Could you check a few things on this model? Use its own coordinates, in mm. Give positions to 0.01 mm unless a question says otherwise; leave off trailing zeros. Write each loop counter-clockwise with the first axis right and the second up, starting at its lowest first coordinate (ties: lowest second). Pieces come first, ordered by that corner, then holes. Notation, with made-up numbers: (-18.5, -23) -> (9.5, -23) arc R16 cw to (9.5, -7) -> close; hole circle Ø2 at (-8.5, 70.5). An arc over 180 degrees is marked (long way). Write item = value, one per line. Start each with the question number.
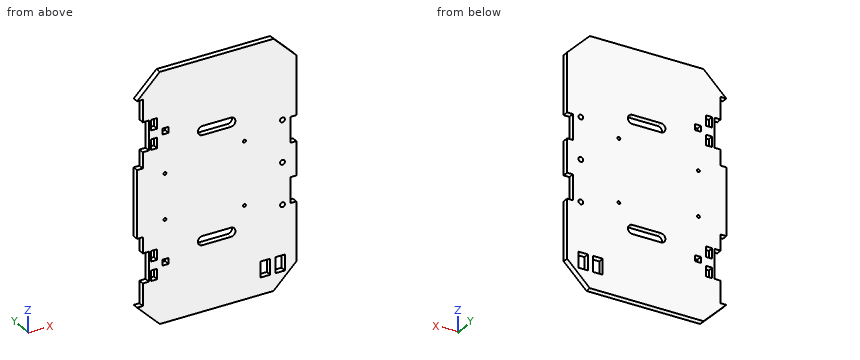
Autodesk Inventor part; units mm, degrees
ref_plane "YZ Plane" through (0, 0, 0) normal (1, 0, 0) x (0, 1, 0)
ref_plane "XZ Plane" through (0, 0, 0) normal (0, 1, 0) x (-1, 0, 0)
ref_plane "XY Plane" through (0, 0, 0) normal (0, 0, 1) x (1, 0, 0)
sketch "Sketch1" plane through (0, 0, 0) normal (0, 1, 0) x (-1, 0, 0)
  line L0 (145, 110) -> (-145, 110)
  line L1 (-145, 110) -> (-145, -110)
  line L2 (-145, -110) -> (145, -110)
  line L3 (145, -110) -> (145, 110)
  line L4 (145, 110) -> (-145, -110) construction
  line L5 (-145, 110) -> (145, -110) construction
  line L6 (105, -80.8333) -> (35, -80.8333)
  line L7 (35, -80.8333) -> (35, -115.8333)
  line L8 (35, -115.8333) -> (105, -115.8333)
  line L9 (105, -115.8333) -> (105, -80.8333)
  line L10 (105, -80.8333) -> (35, -115.8333) construction
  line L11 (35, -80.8333) -> (105, -115.8333) construction
  line L12 (-35, -115.8333) -> (-105, -115.8333)
  line L13 (-105, -115.8333) -> (-105, -80.8333)
  line L14 (-105, -80.8333) -> (-35, -80.8333)
  line L15 (-35, -80.8333) -> (-35, -115.8333)
  line L16 (-35, -115.8333) -> (-105, -80.8333) construction
  line L17 (-105, -115.8333) -> (-35, -80.8333) construction
  line L18 (0, 110) -> (0, -110) construction
  line L19 (5, -110) -> (5, 110)
  point P0 (0, 0)
  point P1 (70, -98.3333)
  point P2 (-70, -98.3333)
  point P3 (0, 0)
  point P4 (-105, -110)
  point P5 (-35, -110)
  point P6 (-15, -80.8333)
  point P7 (-55, -80.8333)
  point P8 (105, -110)
  point P9 (35, -110)
  dimension "d1" = 70
  dimension "d2" = 70
  dimension "d3" = 35
  dimension "d4" = 35
  dimension "d5" = 140
  dimension "d6" = 11.6667
  dimension "d7" = 220
  dimension "d8" = 290
  dimension "d34" = 140
extrude "Extrusion1" add sketch "Sketch1" along normal blind 5 contours L3 L2 L9 L6 L7 L19 L0 | L2 L7 L6 L9
sketch "Sketch5" plane through (0, 5, 0) normal (0, 1, 0) x (1, 0, 0)
  line L0 (-145, -110) -> (-5, -110) construction
  line L1 (-5, -110) -> (-5, 110) construction
  line L2 (-5, 110) -> (-145, 110) construction
  line L3 (-145, 110) -> (-145, -110) construction
  circle A0 centre (-120.5342, 20) radius 1.25
  circle A1 centre (-120.5342, -20) radius 1.25
  circle A2 centre (-50.5342, 28) radius 1.25
  circle A3 centre (-50.5342, -28) radius 1.25
  line L4 (-145, 0) -> (-5, 0) construction
  point P0 (0, 0)
  dimension "d35" = 56
  dimension "d36" = 40
  dimension "d37" = 70
  dimension "d38" = 2.5
  dimension "d39" = 2.5
extrude "Extrusion6" cut sketch "Sketch5" against normal through all
chamfer "Chamfer1" distance 20 angle 45 4 edges at (-145, 2.5, 110) (-145, 2.5, -110) (-5, 2.5, 110) (-5, 2.5, -110)
sketch "Sketch6" plane through (0, 5, 0) normal (0, 1, 0) x (1, 0, 0)
  circle A0 centre (-50.5342, -28) radius 1.25
  circle A1 centre (-50.5342, 28) radius 1.25
  circle A2 centre (-120.5342, -20) radius 1.25
  circle A3 centre (-120.5342, 20) radius 1.25
  line L0 (-25, 110) -> (-5, 90)
  line L1 (-25, 110) -> (-125, 110)
  line L2 (-145, 90) -> (-125, 110)
  line L3 (-145, 90) -> (-145, -90)
  line L4 (-125, -110) -> (-145, -90)
  line L5 (-125, -110) -> (-25, -110)
  line L6 (-5, -90) -> (-25, -110)
  line L7 (-5, -90) -> (-5, 90)
  line L8 (-145, 90) -> (-145, -90)
  line L9 (-5, 37.6) -> (-10, 37.6)
  line L10 (-10, 37.6) -> (-10, 15)
  line L11 (-10, 15) -> (-5, 15)
  line L12 (-5, 15) -> (-5, 37.6)
  line L13 (-5, 37.6) -> (-10, 15) construction
  line L14 (-10, 37.6) -> (-5, 15) construction
  line L15 (-5, -90) -> (-5, 90)
  line L16 (-87.5, 48) -> (-62.5, 48) construction
  line L17 (-87.5, 44) -> (-62.5, 44)
  line L18 (-62.5, 52) -> (-87.5, 52)
  arc A4 (-87.5, 52) -> (-87.5, 44) centre (-87.5, 48) ccw
  arc A5 (-62.5, 44) -> (-62.5, 52) centre (-62.5, 48) ccw
  line L19 (-145, 30) -> (-140, 30)
  line L20 (-140, 30) -> (-140, -30) construction
  line L21 (-140, -30) -> (-145, -30)
  line L22 (-145, -30) -> (-145, 30)
  line L23 (-145, 30) -> (-140, -30) construction
  line L24 (-140, 30) -> (-145, -30) construction
  line L25 (-140, 30) -> (-140, 95)
  line L26 (-140, -30) -> (-140, -95)
  line L27 (-145, 90) -> (-140, 90)
  point P0 (0, 0)
  point P1 (-7.5, 26.3)
  point P2 (-5, 15)
  point P3 (-5, 37.6)
  point P4 (-75, 48)
  point P5 (-75, 110)
  point P6 (-142.5, 0)
  point P7 (-145, 0)
  point P8 (-145, 0)
  dimension "d57" = 5
  dimension "d58" = 22.6
  dimension "d59" = 15
  dimension "d60" = 8
  dimension "d61" = 25
  dimension "d86" = 5
  dimension "d87" = 60
  dimension "d88" = 48
extrude "Extrusion7" cut sketch "Sketch6" against normal through all contours L7 L11 L10 L9 | L27 L25 L19 L3 | A4 L18 A5 L17
mirror "Mirror6" about plane through (0, 0, 0) normal (0, 0, 1) of "Extrusion7"
sketch "Sketch8" plane through (0, 5, 0) normal (0, 1, 0) x (1, 0, 0)
  circle A0 centre (-120.5342, 20) radius 1.25 construction
  circle A1 centre (-120.5342, -20) radius 1.25 construction
  circle A2 centre (-50.5342, 28) radius 1.25 construction
  circle A3 centre (-50.5342, -28) radius 1.25 construction
  line L0 (-87.5, 52) -> (-62.5, 52) construction
  arc A4 (-62.5, 44) -> (-62.5, 52) centre (-62.5, 48) ccw construction
  line L1 (-62.5, 44) -> (-87.5, 44) construction
  arc A5 (-87.5, 52) -> (-87.5, 44) centre (-87.5, 48) ccw construction
  line L2 (-87.5, -44) -> (-62.5, -44) construction
  arc A6 (-62.5, -52) -> (-62.5, -44) centre (-62.5, -48) ccw construction
  line L3 (-62.5, -52) -> (-87.5, -52) construction
  arc A7 (-87.5, -44) -> (-87.5, -52) centre (-87.5, -48) ccw construction
  line L4 (-125, -110) -> (-145, -90) construction
  line L5 (-125, -110) -> (-25, -110) construction
  line L6 (-5, -90) -> (-25, -110) construction
  line L7 (-5, -90) -> (-5, -37.6) construction
  line L8 (-5, -37.6) -> (-10, -37.6) construction
  line L9 (-10, -37.6) -> (-10, -15) construction
  line L10 (-10, -15) -> (-5, -15) construction
  line L11 (-5, -15) -> (-5, 15) construction
  line L12 (-5, 15) -> (-10, 15) construction
  line L13 (-10, 15) -> (-10, 37.6) construction
  line L14 (-10, 37.6) -> (-5, 37.6) construction
  line L15 (-5, 37.6) -> (-5, 90) construction
  line L16 (-25, 110) -> (-5, 90) construction
  line L17 (-25, 110) -> (-125, 110) construction
  line L18 (-145, 90) -> (-125, 110) construction
  line L19 (-145, 30) -> (-145, -30) construction
  line L20 (-23.3, 95) -> (-15, 95)
  line L21 (-15, 95) -> (-15, 81)
  line L22 (-15, 81) -> (-23.3, 81)
  line L23 (-23.3, 81) -> (-23.3, 95)
  line L24 (-23.3, 95) -> (-15, 81) construction
  line L25 (-15, 95) -> (-23.3, 81) construction
  line L26 (-36.3, 95) -> (-28, 95)
  line L27 (-28, 95) -> (-28, 81)
  line L28 (-28, 81) -> (-36.3, 81)
  line L29 (-36.3, 81) -> (-36.3, 95)
  line L30 (-36.3, 95) -> (-28, 81) construction
  line L31 (-28, 95) -> (-36.3, 81) construction
  line L32 (-132.6, -44.1) -> (-127.4, -44.1)
  line L33 (-127.4, -44.1) -> (-127.4, -53.3)
  line L34 (-127.4, -53.3) -> (-132.6, -53.3)
  line L35 (-132.6, -53.3) -> (-132.6, -44.1)
  line L36 (-132.6, -44.1) -> (-127.4, -53.3) construction
  line L37 (-127.4, -44.1) -> (-132.6, -53.3) construction
  line L38 (-132.6, -61.1) -> (-127.4, -61.1)
  line L39 (-127.4, -61.1) -> (-127.4, -70.3)
  line L40 (-127.4, -70.3) -> (-132.6, -70.3)
  line L41 (-132.6, -70.3) -> (-132.6, -61.1)
  line L42 (-132.6, -61.1) -> (-127.4, -70.3) construction
  line L43 (-127.4, -61.1) -> (-132.6, -70.3) construction
  line L44 (-117.4, -54.6) -> (-122.6, -54.6)
  line L45 (-122.6, -54.6) -> (-122.6, -59.8)
  line L46 (-122.6, -59.8) -> (-117.4, -59.8)
  line L47 (-117.4, -59.8) -> (-117.4, -54.6)
  line L48 (-117.4, -54.6) -> (-122.6, -59.8) construction
  line L49 (-122.6, -54.6) -> (-117.4, -59.8) construction
  line L50 (-130, -48.7) -> (-130, -65.7) construction
  line L51 (-140, -44.1) -> (-134.6, -44.1)
  line L52 (-134.6, -44.1) -> (-134.6, -70.3)
  line L53 (-134.6, -70.3) -> (-140, -70.3)
  line L54 (-140, -70.3) -> (-140, -44.1)
  line L55 (-140, -44.1) -> (-134.6, -70.3) construction
  line L56 (-134.6, -44.1) -> (-140, -70.3) construction
  line L57 (-140, 90) -> (-140, 30)
  line L58 (-140, 30) -> (-145, 30)
  line L59 (-145, -30) -> (-140, -30)
  line L60 (-140, -30) -> (-140, -90)
  circle A8 centre (-17.1, 0) radius 2.1
  circle A9 centre (-17.1, 37) radius 2.1
  circle A10 centre (-17.1, -37) radius 2.1
  point P0 (0, 0)
  point P1 (-19.15, 88)
  point P2 (-32.15, 88)
  point P3 (-120, -57.2)
  point P4 (-130, -57.2)
  point P5 (-137.3, -57.2)
  point P6 (-140, 95)
  point P7 (-140, -95)
  dimension "d63" = 14
  dimension "d64" = 8.3
  dimension "d65" = 14
  dimension "d66" = 8.3
  dimension "d67" = 13
  dimension "d68" = 15
  dimension "d69" = 10
  dimension "d72" = 52.8
  dimension "d73" = 10
  dimension "d74" = 9.2
  dimension "d75" = 9.2
  dimension "d76" = 5.2
  dimension "d77" = 5.2
  dimension "d78" = 5.2
  dimension "d79" = 5.2
  dimension "d80" = 15
  dimension "d81" = 17
  dimension "d83" = 2
  dimension "d89" = 4.2
  dimension "d90" = 4.2
  dimension "d91" = 4.2
  dimension "d92" = 17.1
  dimension "d93" = 37
  dimension "d94" = 37
extrude "Extrusion8" cut sketch "Sketch8" against normal through all contours L20 L21 L22 L23 | L26 L27 L28 L29 | A8 | A9 | A10
extrude "Extrusion9" cut sketch "Sketch8" against normal through all contours L32 L33 L34 L35 | L38 L39 L40 L41 | L47 L46 L45 L44 | L51 L52 L53 L54
mirror "Mirror7" about plane through (0, 0, 0) normal (0, 0, 1) of "Extrusion9"
equation "\"d2\" = d1"
equation "\"d4\" = d3"
equation "\"d39\" = d38"
equation "\"d65\" = d63"
equation "\"d66\" = d64"
equation "\"d75\" = d74"
equation "\"d77\" = d76"
equation "\"d90\" = d89"
equation "\"d91\" = d89"
equation "\"d94\" = d93"
properties part number "top-plate"
(1) If I drill on line 1 along Z through (x, y) = (-71.5, 1.6); line 2 along Z through (x, y) = (-17.1, 2.9); line 3 along X through (y, z) = (3.5, 37), over which ranges is the centre line in solid material (lowest first)? Write a range as from..to.
(2) Imagine slicing it at B-B (x = -17.1). Please give me the cut outline in (y, z).
(3) I'm going to push flat-ended pins straight in: pin 1 (2.5 mm diameter, centred on x = -131, y = 3, fed in from -Z); pin 2 (8 mm diameter, centred on x = -57, z = 45.5, fed in from -Y); pin 3 (1.5 mm diameter, centred on x = -138.5, y = 2.5, fed in from -Z); pin 4 (2.5 mm diameter, centred on y = 3.5, z = -26, fed in from +X). Where does each tip first touch, or does it pass through?
(4) Imagine slicing it at D-D (x = -79). Please give me the cut outline in (y, z), then the cut area to 3 significant figures.
(5) Imagine slicing it at C-C (z = 0). Please give me the cut outline in (x, y), then the cut area to 3 significant figures.
(6) Imagine slicing it at A-A (z = -48). Please give me the cut outline in (x, y).
Answers below:
q1.line_1 = -110..-52, -44..44, 52..110
q1.line_2 = -102.1..-95, -81..-39.1, -34.9..-2.1, 2.1..34.9, 39.1..102.1
q1.line_3 = -140..-19.2, -15..-10
q2.outline = (0, -102.1) -> (5, -102.1) -> (5, -95) -> (0, -95) -> close; (0, -81) -> (5, -81) -> (5, -39.1) -> (0, -39.1) -> close; (0, -34.9) -> (5, -34.9) -> (5, -2.1) -> (0, -2.1) -> close; (0, 2.1) -> (5, 2.1) -> (5, 34.9) -> (0, 34.9) -> close; (0, 39.1) -> (5, 39.1) -> (5, 102.1) -> (0, 102.1) -> close
q3.pin_1 = -105.25
q3.pin_2 = 0
q3.pin_3 = -97.25
q3.pin_4 = -10
q4.outline = (0, -110) -> (5, -110) -> (5, -52) -> (0, -52) -> close; (0, -44) -> (5, -44) -> (5, 44) -> (0, 44) -> close; (0, 52) -> (5, 52) -> (5, 110) -> (0, 110) -> close
q4.area = 1,020 mm^2
q5.outline = (-145, 0) -> (-19.2, 0) -> (-19.2, 5) -> (-145, 5) -> close; (-15, 0) -> (-5, 0) -> (-5, 5) -> (-15, 5) -> close
q5.area = 679 mm^2
q6.outline = (-134.6, 0) -> (-132.6, 0) -> (-132.6, 5) -> (-134.6, 5) -> close; (-127.4, 0) -> (-91.5, 0) -> (-91.5, 5) -> (-127.4, 5) -> close; (-58.5, 0) -> (-5, 0) -> (-5, 5) -> (-58.5, 5) -> close
